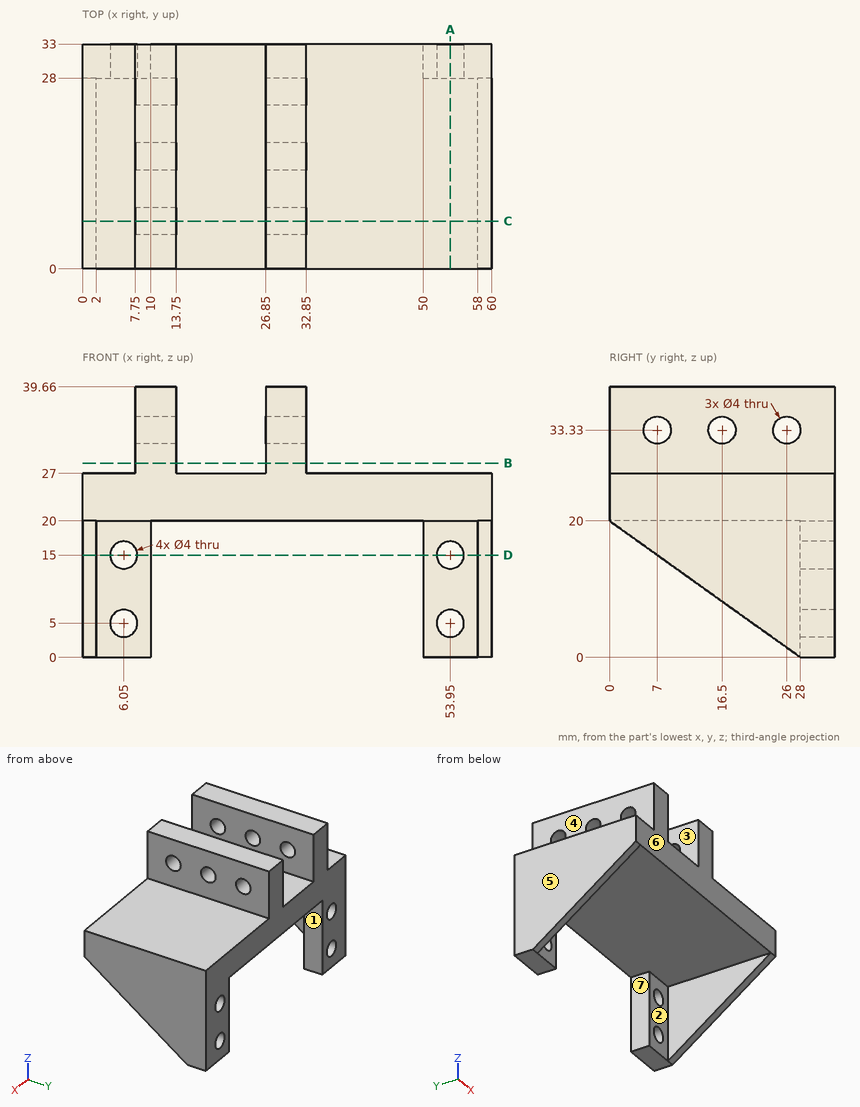
Could you check a few things on this drawing? It's one solid part, dimensions in mm from its lowest x, y, z. A direction names the side the tool comes from. Round coordinates to 2 decimals unless told otherwise and drop trailing zeros. Loops run counter-clockwise (first coordinate to the right, second up) from the corner with the lowest first, then second, coordinate; pieces in that order, holes last. Notation, with made-up numbers: M 4.5,66 L 24.5,66 A23 cw 24.5,89 Z; hole C 20,71 d3. An arc over 180 degrees is marked long. Write each question's results on one line, items separated by ' | '. Start each with the question number.
(1) Will these pins go through, and if not, where does the flat tip stop? P1, Ø6.5, axis at y = 26, z = 33.33, coming from the +X side; P2, Ø6.5, axis at x = 7, z = 13, coming from the -Y side; P3, Ø12, axis at x = 45.5, y = 23.5, coming from the +Z side.
(2) Thinking about a two-plate mould opening in X: for the marked faces 5, 6 and 7, which applies, pulls with the +X half, pulls with the -X half, needs draft (parallel to the pull), parting line crosses it, or undercut?
(3) If I drill on probe 1 along X at (y, z) = (29.55, 15); probe 2 along Y at (x, z) = (10.55, 33.33); probe 3 along Y at (x, z) = (12, 34), over which ranges is the centre line in solid material (lowest first)? Write a range as from..to.
(4) I want a section at B-B (z = 28.5). Please give me the cut outline in (x, y).
(5) I want a section at A-A (x = 53.95). Please give me the cut outline in (y, z).
(6) On a 3-axis mill with a long thin cutter (end or side, diameter ignored), from which of +Z, -Z, +X, -X, +Y, -Y can I reach the whole of each face in a straight line? I mean the marked faces 1, 2, 3 and 4. Say none if no direction works.
(7) I want a section at D-D (z = 15). Please give me the cut outline in (x, y), then the cut area to 3 significant figures.
(8) I want a section at C-C (y = 7). Please give me the cut outline in (x, z), then the cut area to 3 significant figures.
Solved:
1) P1: stops at x = 32.85 | P2: stops at y = 28 | P3: stops at z = 27
2) face 5: pulls with the -X half | face 6: needs draft | face 7: undercut
3) probe 1: x = 0..4.05, 8.05..10, 50..51.95, 55.95..60 | probe 2: y = 0..5, 9..14.5, 18.5..24, 28..33 | probe 3: y = 0..5.12, 8.88..14.62, 18.38..24.12, 27.88..33
4) outline: M 7.75,0 L 13.75,0 L 13.75,33 L 7.75,33 Z; M 26.85,0 L 32.85,0 L 32.85,33 L 26.85,33 Z
5) outline: M 0,20 L 28,20 L 28,17 L 33,17 L 33,27 L 0,27 Z; M 28,0 L 33,0 L 33,3 L 28,3 Z; M 28,7 L 33,7 L 33,13 L 28,13 Z
6) face 1: -Z, +Y, -Y | face 2: -Z, -Y | face 3: +Z, +Y, -Y | face 4: +Z, -X, +Y, -Y
7) outline: M 0,7 L 2,7 L 2,28 L 4.05,28 L 4.05,33 L 0,33 Z; M 8.05,28 L 10,28 L 10,33 L 8.05,33 Z; M 50,28 L 51.95,28 L 51.95,33 L 50,33 Z; M 55.95,28 L 58,28 L 58,7 L 60,7 L 60,33 L 55.95,33 Z | area: 144 mm²
8) outline: M 0,15 L 2,15 L 2,20 L 58,20 L 58,15 L 60,15 L 60,27 L 32.85,27 L 32.85,31.33 L 26.85,31.33 L 26.85,27 L 13.75,27 L 13.75,31.33 L 7.75,31.33 L 7.75,27 L 0,27 Z; M 7.75,35.33 L 13.75,35.33 L 13.75,39.66 L 7.75,39.66 Z; M 26.85,35.33 L 32.85,35.33 L 32.85,39.66 L 26.85,39.66 Z | area: 544 mm²
